Input: part model. Units: mm. Frame: model coordinates. A direction names the side the tool comes from. Round coordinates to 2 decimals unless told otherwise and drop trailing zeros. Loops run counter-clockwise (first coordinate to the right, second up) from the corner with the lowest first, then second, coordinate; pieces in that order, holes last. Notation, with made-up numbers: (31, -11.5) - (43, -11.5) arc R29 ccw to (43, 14.5) - close; hole circle Ø2 at (74.25, 70.5). An arc over 180 degrees is marked (long way). Write each question's results on one line, items separated by ' | '.
from build123d import *

# Parameters (mm, degrees)
PAD002_DEPTH = 20


with BuildPart() as part:
    # Sketch002 → Pad002 (new body)
    with BuildSketch(Plane.XY):
        with BuildLine():
            Line((11.462484, 11.058947), (334.462484, 11.058947))
            ThreePointArc((340.462484, 5.058947), (338.705124, 9.301588), (334.462484, 11.058947))
            Line((340.462484, 5.058947), (340.462484, -355.941053))
            ThreePointArc((334.462484, -361.941053), (338.705124, -360.183694), (340.462484, -355.941053))
            Line((334.462484, -361.941053), (11.462484, -361.941053))
            ThreePointArc((5.462484, -355.941053), (7.219843, -360.183694), (11.462484, -361.941053))
            Line((5.462484, -355.941053), (5.462484, 5.058947))
            ThreePointArc((11.462484, 11.058947), (7.219843, 9.301588), (5.462484, 5.058947))
        make_face()
        with BuildLine():
            Line((78.462484, -38.941053), (267.462484, -38.941053))
            ThreePointArc((270.462484, -41.941053), (269.583804, -39.819733), (267.462484, -38.941053))
            Line((270.462484, -41.941053), (270.462484, -106.941053))
            ThreePointArc((267.462484, -109.941053), (269.583804, -109.062373), (270.462484, -106.941053))
            Line((267.462484, -109.941053), (78.462484, -109.941053))
            ThreePointArc((75.462484, -106.941053), (76.341163, -109.062373), (78.462484, -109.941053))
            Line((75.462484, -106.941053), (75.462484, -41.941053))
            ThreePointArc((78.462484, -38.941053), (76.341163, -39.819733), (75.462484, -41.941053))
        make_face(mode=Mode.SUBTRACT)
        with BuildLine():
            Line((78.462484, -139.941053), (267.462484, -139.941053))
            ThreePointArc((270.462484, -142.941053), (269.583804, -140.819733), (267.462484, -139.941053))
            Line((270.462484, -142.941053), (270.462484, -207.941053))
            ThreePointArc((267.462484, -210.941053), (269.583804, -210.062373), (270.462484, -207.941053))
            Line((267.462484, -210.941053), (78.462484, -210.941053))
            ThreePointArc((75.462484, -207.941053), (76.341163, -210.062373), (78.462484, -210.941053))
            Line((75.462484, -207.941053), (75.462484, -142.941053))
            ThreePointArc((78.462484, -139.941053), (76.341163, -140.819733), (75.462484, -142.941053))
        make_face(mode=Mode.SUBTRACT)
        with BuildLine():
            Line((78.462484, -240.941053), (267.462484, -240.941053))
            ThreePointArc((270.462484, -243.941053), (269.583804, -241.819733), (267.462484, -240.941053))
            Line((270.462484, -243.941053), (270.462484, -308.941053))
            ThreePointArc((267.462484, -311.941053), (269.583804, -311.062373), (270.462484, -308.941053))
            Line((267.462484, -311.941053), (78.462484, -311.941053))
            ThreePointArc((75.462484, -308.941053), (76.341163, -311.062373), (78.462484, -311.941053))
            Line((75.462484, -308.941053), (75.462484, -243.941053))
            ThreePointArc((78.462484, -240.941053), (76.341163, -241.819733), (75.462484, -243.941053))
        make_face(mode=Mode.SUBTRACT)
    extrude(amount=-PAD002_DEPTH)


solid = part.part
1. Section query A-A, the plane y = -102.5. Output: boundary loops of the cut face in (x, z), plus the area to 3 significant figures.
Answer:
outline: (5.46, -20) - (75.46, -20) - (75.46, 0) - (5.46, 0) - close; (270.46, -20) - (340.46, -20) - (340.46, 0) - (270.46, 0) - close | area: 2,800 mm^2
2. Set-up query: faces 5 (the flat face through (171, 11.059, -10)), 6 (the flat face through (174, -109.941, -10)). Return all of +Z, -Z, +X, -X, +Y, -Y with unobstructed straight access to the full face (end or side cutting, diameter ignored); none if empty.
Answer:
face 5: +Z, -Z, +X, -X, +Y | face 6: +Z, -Z
3. Mould query, pull axis X, two halves, no side actions, for faces 1 (the flat face through (172, -38.941, -10)), 2 (the flat face through (174, -311.941, -10)), 3 (the flat face through (175, -214, 0)), 4 (the flat face through (340.462, -173, -10)). Classes: pulls with the +X half, pulls with the -X half, needs draft (parallel to the pull), parting line crosses it, or undercut.
Answer:
face 1: undercut | face 2: undercut | face 3: needs draft | face 4: pulls with the +X half
4. Line query: line 1 (Y direction, x = 80, z = -15); line 2 (X direction, y = -62, z = -5); line 3 (X direction, y = -210, z = -5.25). Output: solid intervals per line, ascending. Write a range as [from, to].
Answer:
line 1: [-361.94, -311.94], [-240.94, -210.94], [-139.94, -109.94], [-38.94, 11.06] | line 2: [5.46, 75.46], [270.46, 340.46] | line 3: [5.46, 76.28], [269.64, 340.46]
5. Section query B-B, the plane x = 187.5. Output: boundary loops of the cut face in (y, z).
Answer:
outline: (-361.94, -20) - (-311.94, -20) - (-311.94, 0) - (-361.94, 0) - close; (-240.94, -20) - (-210.94, -20) - (-210.94, 0) - (-240.94, 0) - close; (-139.94, -20) - (-109.94, -20) - (-109.94, 0) - (-139.94, 0) - close; (-38.94, -20) - (11.06, -20) - (11.06, 0) - (-38.94, 0) - close
6. Section query C-C, the plane z = -4.25. Count the separate pieces of the cut face and the enclosed holes in it, plus the area to 3 significant figures.
Answer:
separate pieces: 1 | enclosed holes: 3 | area: 83,400 mm^2
